Geometry: see drawing. Coordinates: mm, zero at the bounding-box minimum. A direction names the side the tool comes from. Round coordinates to 2 decimals unless told otherwise and drop trailing zeros. Order: outer loops, then holes, each group sorted by start corner. A loop starts at its lowest first (then second) coordinate and runs counter-clockwise, first axis right, second up. Notation, with made-up numbers: M -15.75,27 L 28.25,27 A19 ccw 28.25,31 Z; hole C 12,-36.5 d1. An arc over 180 degrees is marked long. Answer in a Markdown table with one row per item. Add a question column.
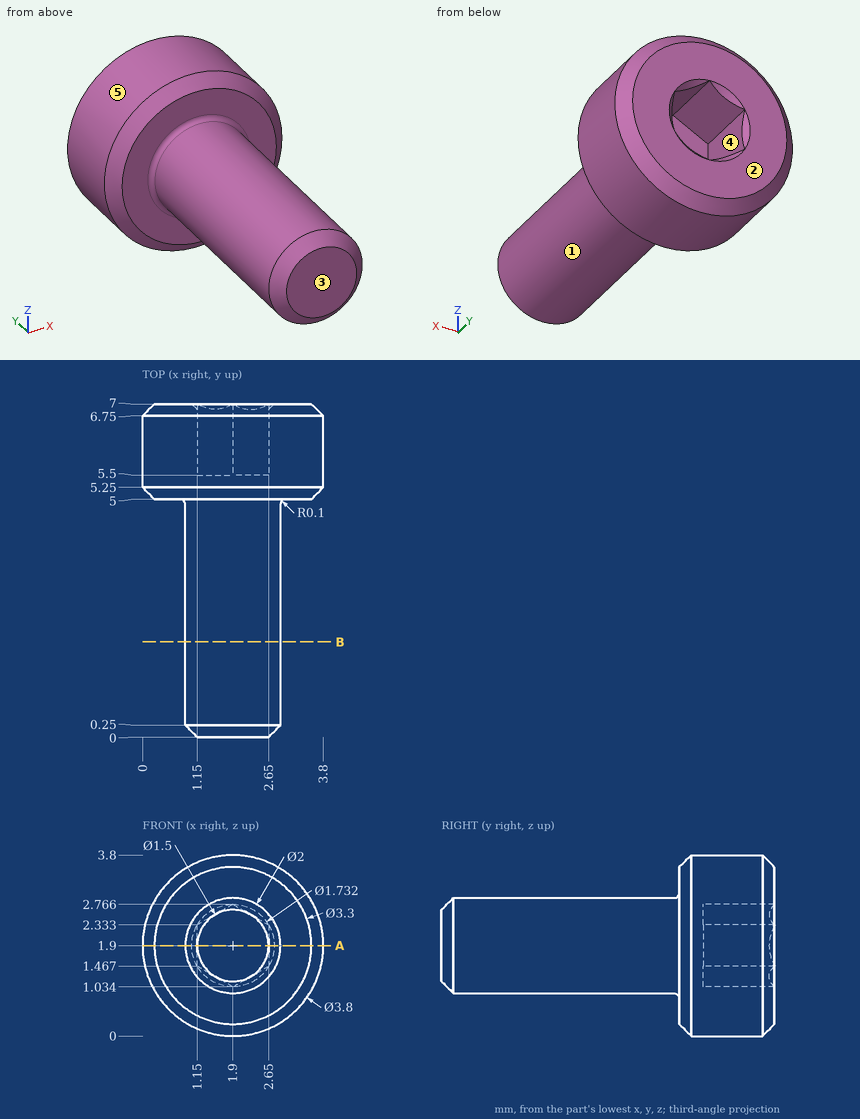
(1) Draft query along Z for the marked faces 3, 4 and 5. Return one class per face: +Z half, -Z half, draft (parallel to the pull), parting line (faces both ways), or undercut.
(2) Cut plane B-B (y = 2). Return loops of the section in (x, z), and give its area (3 significant figures).
(3) Access query for the marked faces 1 and 2. Directions: +Z, -Z, +X, -X, +Y, -Y. A direction counts if a zero-diameter tool reaches every point of the face in a straight line with its end or side. Return the directions, or none.
(4) Cut plane A-A (z = 1.9). Return loops of the section in (x, y), and give its area (3 significant figures).
(5) Pin query (flat end, axial travel): pin 1 (1 mm diameter, centred on y = 5.5, z = 3, fed in from +X); pin 2 (1.5 mm diameter, centred on x = 3.5, y = 6, fed in from +Z). Return the tip coordinate at first contact, or that it passes through.
(6) Line query: line 1 (X direction, y = 4.5, z = 1.4); line 2 (Y direction, x = 2.3, z = 2.5); line 3 (Y direction, x = 1.75, z = 3.2). Output: solid intervals per line, ascending. Write a range as from..to.
Answer list:
| question | item | result |
|---|---|---|
| 1 | face 3 | draft |
| 1 | face 4 | undercut |
| 1 | face 5 | parting line |
| 2 | outline | C 1.9,1.9 d2 |
| 2 | area | 3.14 mm² |
| 3 | face 1 | -Y |
| 3 | face 2 | +Z, -Z, +X, -X, +Y |
| 4 | outline | M 0,5.25 L 0.25,5 L 0.8,5 A0.1 cw 0.9,4.9 L 0.9,0.25 L 1.15,0 L 2.65,0 L 2.9,0.25 L 2.9,4.9 A0.1 cw 3,5 L 3.55,5 L 3.8,5.25 L 3.8,6.75 L 3.55,7 L 2.77,7 L 2.65,6.88 L 2.65,5.5 L 1.15,5.5 L 1.15,6.88 L 1.03,7 L 0.25,7 L 0,6.75 Z |
| 4 | area | 15.2 mm² |
| 5 | pin 1 | x = 3.7 |
| 5 | pin 2 | z = 3.6 |
| 6 | line 1 | 1.03..2.77 |
| 6 | line 2 | 0..5.5 |
| 6 | line 3 | 5..7 |
